from build123d import *

# Parameters (mm, degrees)
F0_W     = 127
F0_H     = 127
F2_DEPTH = 12.7


# Not quite as in the source:
# - the program builds the solid bodies; features that only make, move or delete a surface that nothing else refers to are left out


with BuildPart() as f2:
    # F0 (on Top) → F2 (new body)
    with BuildSketch(Plane.XY):
        Rectangle(F0_W, F0_H)
        with BuildLine():
            ThreePointArc((-50.8, 45.085), (-54.8411152545, 54.8411152545), (-45.085, 50.8))
            Line((-45.085, 50.8), (45.085, 50.8))
            ThreePointArc((45.085, 50.8), (50.8, 56.515), (56.515, 50.8))
            ThreePointArc((56.515, 50.8), (54.8411152545, 46.7588847455), (50.8, 45.085))
            Line((50.8, 45.085), (50.8, -45.085))
            ThreePointArc((50.8, -45.085), (54.8411152545, -46.7588847455), (56.515, -50.8))
            ThreePointArc((56.515, -50.8), (50.8, -56.515), (45.085, -50.8))
            Line((45.085, -50.8), (-45.085, -50.8))
            ThreePointArc((-45.085, -50.8), (-54.8411152545, -54.8411152545), (-50.8, -45.085))
            Line((-50.8, -45.085), (-50.8, 45.085))
        make_face(mode=Mode.SUBTRACT)
        with BuildLine():
            Line((45.085, 50.8), (-45.085, 50.8))
            ThreePointArc((-45.085, 50.8), (-46.7588847455, 46.7588847455), (-50.8, 45.085))
            Line((-50.8, 45.085), (-50.8, -45.085))
            ThreePointArc((-50.8, -45.085), (-46.7588847455, -46.7588847455), (-45.085, -50.8))
            Line((-45.085, -50.8), (45.085, -50.8))
            ThreePointArc((45.085, -50.8), (46.7588847455, -46.7588847455), (50.8, -45.085))
            Line((50.8, -45.085), (50.8, 45.085))
            ThreePointArc((50.8, 45.085), (46.7588847455, 46.7588847455), (45.085, 50.8))
        make_face()
    extrude(amount=F2_DEPTH)


solid = f2.part
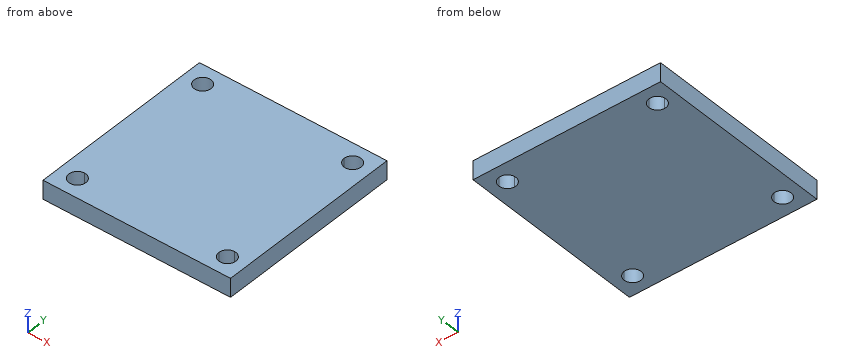
Input: part model. Units: mm. Frame: model coordinates. Give positions to 0.01 mm unless a question says otherwise; leave off trailing zeros. Write each loop counter-clockwise with the first axis right and the second up, starting at its lowest first coordinate (ties: lowest second). Pieces come first, ordered by that corner, then holes. Notation, with made-up numbers: M 53.25,-1.5 L 92.25,-1.5 A14 cw 92.25,15.5 Z; hole C -5.75,-16 d11. An arc over 180 degrees is marked long. Use one line per item in the form item = value.
1. Cut plane A-A on z = 7.25. Return loops of the section in (x, y) (3 decimals), and give its area (3 significant figures).
Outcome:
outline = M -63.5,-63.5 L 63.5,-63.5 L 63.5,63.5 L -63.5,63.5 Z; hole C -50.8,-50.8 d11.43; hole C -50.8,50.8 d11.43; hole C 50.8,-50.8 d11.43; hole C 50.8,50.8 d11.43
area = 15,700 mm²
2. First-contact query: P1, Ø10, axis at x = -4, y = 13.5, coming from the -Z side. Flat tip, straight axial feed; report the tip coordinate or a pass-through.
Outcome:
P1 = 0
3. Cut plane B-B on y = -53.5. Return loops of the section in (x, z), and give its area (3 significant figures).
Outcome:
outline = M -63.5,0 L -55.84,0 L -55.84,12.7 L -63.5,12.7 Z; M -45.76,0 L 45.76,0 L 45.76,12.7 L -45.76,12.7 Z; M 55.84,0 L 63.5,0 L 63.5,12.7 L 55.84,12.7 Z
area = 1,360 mm²
4. Ray query, L1, parallel to X at y = -50.8, z = 7.25 (3 decimals); L2, parallel to Y at x = 54, z = 12. Return the intervals inside material, ascending.
Outcome:
L1 = -63.5 to -56.515, -45.085 to 45.085, 56.515 to 63.5
L2 = -63.5 to -55.54, -46.06 to 46.06, 55.54 to 63.5
